```python
from build123d import *

# Parameters (mm, degrees)
SKETCH1_R           = 2.6035
BOSS_EXTRUDE1_DEPTH = 69.85


with BuildPart() as part:
    # Sketch1 → Boss-Extrude1 (new body)
    with BuildSketch(Plane(origin=(0, 0, 0), x_dir=(0, 0, -1), z_dir=(1, 0, 0))):
        with BuildLine():
            Line((6.333126718, -12.7), (9.550443118, -12.7))
            ThreePointArc((9.550443118, -12.7), (10.058366869, -12.192000006), (10.566443095, -12.699847501))
            ThreePointArc((10.566443095, -12.699847501), (12.082537762, -12.08250727), (12.699846982, -10.566399977))
            ThreePointArc((12.699846982, -10.566399977), (12.192000006, -10.058323491), (12.7, -9.5504))
            Line((12.7, -9.5504), (12.7, -6.3330836))
            ThreePointArc((12.7, -6.3330836), (12.192, -5.8250836), (12.7, -5.3170836))
            Line((12.7, -5.3170836), (12.7, -4.287469289))
            ThreePointArc((12.7, -4.287469289), (12.39275138, -3.545705502), (11.650987593, -3.238456882))
            Line((11.650987593, -3.238456882), (11.539212407, -3.238456882))
            ThreePointArc((11.539212407, -3.238456882), (10.79744862, -3.545705502), (10.4902, -4.287469289))
            Line((10.4902, -4.287469289), (10.4902, -6.402089023))
            ThreePointArc((10.4902, -6.402089023), (9.856505071, -7.351067942), (8.737131347, -7.129408934))
            Line((8.737131347, -7.129408934), (4.5085, -2.9104418))
            Line((4.5085, -2.9104418), (4.5085, 1.593185507))
            ThreePointArc((4.5085, 1.593185507), (4.750877967, 2.809883091), (5.441005833, 3.840816462))
            Line((5.441005833, 3.840816462), (8.737131347, 7.129408934))
            ThreePointArc((8.737131347, 7.129408934), (9.856505071, 7.351067942), (10.4902, 6.402089023))
            Line((10.4902, 6.402089023), (10.4902, 4.287469289))
            ThreePointArc((10.4902, 4.287469289), (10.79744862, 3.545705502), (11.539212407, 3.238456882))
            Line((11.539212407, 3.238456882), (11.650987593, 3.238456882))
            ThreePointArc((11.650987593, 3.238456882), (12.39275138, 3.545705502), (12.7, 4.287469289))
            Line((12.7, 4.287469289), (12.7, 5.3170836))
            ThreePointArc((12.7, 5.3170836), (12.192, 5.8250836), (12.7, 6.3330836))
            Line((12.7, 6.3330836), (12.7, 9.5504))
            ThreePointArc((12.7, 9.5504), (12.192000006, 10.058323491), (12.699846982, 10.566399977))
            ThreePointArc((12.699846982, 10.566399977), (12.082537762, 12.08250727), (10.566443095, 12.699847501))
            ThreePointArc((10.566443095, 12.699847501), (10.058366869, 12.192000006), (9.550443118, 12.7))
            Line((9.550443118, 12.7), (6.333126718, 12.7))
            ThreePointArc((6.333126718, 12.7), (5.825126718, 12.192), (5.317126718, 12.7))
            Line((5.317126718, 12.7), (4.287512407, 12.7))
            ThreePointArc((4.287512407, 12.7), (3.54574862, 12.39275138), (3.2385, 11.650987593))
            Line((3.2385, 11.650987593), (3.2385, 11.539212407))
            ThreePointArc((3.2385, 11.539212407), (3.54574862, 10.79744862), (4.287512407, 10.4902))
            Line((4.287512407, 10.4902), (6.476788598, 10.4902))
            ThreePointArc((6.476788598, 10.4902), (7.432222385, 9.85140422), (7.207036008, 8.724370562))
            Line((7.207036008, 8.724370562), (3.898272566, 5.423169045))
            ThreePointArc((3.898272566, 5.423169045), (2.869120213, 4.736787962), (1.655778399, 4.4958))
            Line((1.655778399, 4.4958), (-1.655778399, 4.4958))
            ThreePointArc((-1.655778399, 4.4958), (-2.869120213, 4.736787962), (-3.898272566, 5.423169045))
            Line((-3.898272566, 5.423169045), (-7.207036008, 8.724370562))
            ThreePointArc((-7.207036008, 8.724370562), (-7.432222385, 9.85140422), (-6.476788598, 10.4902))
            Line((-6.476788598, 10.4902), (-4.287512407, 10.4902))
            ThreePointArc((-4.287512407, 10.4902), (-3.54574862, 10.79744862), (-3.2385, 11.539212407))
            Line((-3.2385, 11.539212407), (-3.2385, 11.650987593))
            ThreePointArc((-3.2385, 11.650987593), (-3.54574862, 12.39275138), (-4.287512407, 12.7))
            Line((-4.287512407, 12.7), (-5.317126718, 12.7))
            ThreePointArc((-5.317126718, 12.7), (-5.825126718, 12.192), (-6.333126718, 12.7))
            Line((-6.333126718, 12.7), (-9.550443118, 12.7))
            ThreePointArc((-9.550443118, 12.7), (-10.058366869, 12.192000006), (-10.566443095, 12.699847501))
            ThreePointArc((-10.566443095, 12.699847501), (-12.082537762, 12.08250727), (-12.699846982, 10.566399977))
            ThreePointArc((-12.699846982, 10.566399977), (-12.192000006, 10.058323491), (-12.7, 9.5504))
            Line((-12.7, 9.5504), (-12.7, 6.3330836))
            ThreePointArc((-12.7, 6.3330836), (-12.192, 5.8250836), (-12.7, 5.3170836))
            Line((-12.7, 5.3170836), (-12.7, 4.287469289))
            ThreePointArc((-12.7, 4.287469289), (-12.39275138, 3.545705502), (-11.650987593, 3.238456882))
            Line((-11.650987593, 3.238456882), (-11.539212407, 3.238456882))
            ThreePointArc((-11.539212407, 3.238456882), (-10.79744862, 3.545705502), (-10.4902, 4.287469289))
            Line((-10.4902, 4.287469289), (-10.4902, 6.402089023))
            ThreePointArc((-10.4902, 6.402089023), (-9.856505071, 7.351067942), (-8.737131347, 7.129408934))
            Line((-8.737131347, 7.129408934), (-5.441005833, 3.840816462))
            ThreePointArc((-5.441005833, 3.840816462), (-4.750877967, 2.809883091), (-4.5085, 1.593185507))
            Line((-4.5085, 1.593185507), (-4.5085, -1.593185507))
            ThreePointArc((-4.5085, -1.593185507), (-4.750877967, -2.809883091), (-5.441005833, -3.840816462))
            Line((-5.441005833, -3.840816462), (-8.737131347, -7.129408934))
            ThreePointArc((-8.737131347, -7.129408934), (-9.856505071, -7.351067942), (-10.4902, -6.402089023))
            Line((-10.4902, -6.402089023), (-10.4902, -4.287469289))
            ThreePointArc((-10.4902, -4.287469289), (-10.79744862, -3.545705502), (-11.539212407, -3.238456882))
            Line((-11.539212407, -3.238456882), (-11.650987593, -3.238456882))
            ThreePointArc((-11.650987593, -3.238456882), (-12.39275138, -3.545705502), (-12.7, -4.287469289))
            Line((-12.7, -4.287469289), (-12.7, -5.3170836))
            ThreePointArc((-12.7, -5.3170836), (-12.192, -5.8250836), (-12.7, -6.3330836))
            Line((-12.7, -6.3330836), (-12.7, -9.5504))
            ThreePointArc((-12.7, -9.5504), (-12.192000006, -10.058323491), (-12.699846982, -10.566399977))
            ThreePointArc((-12.699846982, -10.566399977), (-12.082537762, -12.08250727), (-10.566443095, -12.699847501))
            ThreePointArc((-10.566443095, -12.699847501), (-10.058366869, -12.192000006), (-9.550443118, -12.7))
            Line((-9.550443118, -12.7), (-6.333126718, -12.7))
            ThreePointArc((-6.333126718, -12.7), (-5.825126718, -12.192), (-5.317126718, -12.7))
            Line((-5.317126718, -12.7), (-4.287512407, -12.7))
            ThreePointArc((-4.287512407, -12.7), (-3.54574862, -12.39275138), (-3.2385, -11.650987593))
            Line((-3.2385, -11.650987593), (-3.2385, -11.539212407))
            ThreePointArc((-3.2385, -11.539212407), (-3.54574862, -10.79744862), (-4.287512407, -10.4902))
            Line((-4.287512407, -10.4902), (-6.416408329, -10.4902))
            ThreePointArc((-6.416408329, -10.4902), (-7.41473083, -9.822813117), (-7.179650497, -8.645192506))
            Line((-7.179650497, -8.645192506), (-3.952270251, -5.423690499))
            ThreePointArc((-3.952270251, -5.423690499), (-2.922936451, -4.736929036), (-1.709253557, -4.4958))
            Line((-1.709253557, -4.4958), (1.709253557, -4.4958))
            ThreePointArc((1.709253557, -4.4958), (2.922936451, -4.736929036), (3.952270251, -5.423690499))
            Line((3.952270251, -5.423690499), (7.179650497, -8.645192506))
            ThreePointArc((7.179650497, -8.645192506), (7.41473083, -9.822813117), (6.416408329, -10.4902))
            Line((6.416408329, -10.4902), (4.287512407, -10.4902))
            ThreePointArc((4.287512407, -10.4902), (3.54574862, -10.79744862), (3.2385, -11.539212407))
            Line((3.2385, -11.539212407), (3.2385, -11.650987593))
            ThreePointArc((3.2385, -11.650987593), (3.54574862, -12.39275138), (4.287512407, -12.7))
            Line((4.287512407, -12.7), (5.317126718, -12.7))
            ThreePointArc((5.317126718, -12.7), (5.825126718, -12.192), (6.333126718, -12.7))
        make_face()
        Circle(SKETCH1_R, mode=Mode.SUBTRACT)
    extrude(amount=BOSS_EXTRUDE1_DEPTH)


solid = part.part
```
Work out the finished part from the listing and answer in its coordinate system (mm). A direction names the side the tool comes from. Give positions to 0.01 mm unless a question says otherwise; leave off trailing zeros. Loops run counter-clockwise (first coordinate to the right, second up) from the corner with the lowest first, then second, coordinate; pieces in that order, holes last. Notation, with made-up numbers: (58.5, -19.5) -> (110.5, -19.5) arc R36 ccw to (110.5, 15.5) -> close; hole circle Ø9 at (-1, -24.5). An arc over 180 degrees is marked (long way). Write item = value, one per line. Start each with the question number.
(1) Find section A-A on z = 0. Give the vertices of the cut face in (x, y).
(2) Find the intervals of material crossed by probe 1 along Y at (x, z) = (6.5, 2); probe 2 along Y at (x, z) = (48.5, -8.75); probe 3 along Z at (x, y) = (22.5, -9), in increasing order. Write a range as from..to.
(3) The mould has two halves that part along Z. Classify faces 3 (the flat face through (34, 8, -12.7)), 4 (the cylindrical face through (34.436, 7.344, 9.872)), 5 (the flat face through (34, 8, 12.7)): +Z half, -Z half, draft (parallel to the pull), parting line (faces both ways), or undercut.
(4) Find section B-B on y = 0. Give the vertices of the cut face in (x, z), and give its area (3 significant figures).
(5) Given pin 1 Ø0.6 at (x, y) = (35, 5.5) entering from -Z; pin 2 Ø1.4 at (x, y) = (52.5, -1.5) entering from -Z; pin 3 Ø2 at (x, y) = (14.5, 1) entering from +Z; pin 4 Ø1.7 at (x, z) = (48.5, 0.5) entering from +Y, each flat-ended and moving along its own axis, determine where each tip first touches the part or whether it passes through.
(6) Which of the six approach directions +Z, -Z, +X, -X, +Y, -Y give full straight-line access (tool end or side, diameter ignored) to faces 1 (the flat face through (34, 12.7, -8)), 2 (the flat face through (34, -10.49, -5))?
From the geometry:
q1.outline = (0, -4.5) -> (69.85, -4.5) -> (69.85, -2.6) -> (0, -2.6) -> close; (0, 2.6) -> (69.85, 2.6) -> (69.85, 4.5) -> (0, 4.5) -> close
q2.probe_1 = -4.51..-1.67, 1.67..4.51
q2.probe_2 = -12.7..-7.14, 7.14..12.7
q2.probe_3 = -12.7..-7.42, 7.42..12.7
q3.face_3 = -Z half
q3.face_4 = undercut
q3.face_5 = +Z half
q4.outline = (0, -4.51) -> (69.85, -4.51) -> (69.85, -2.6) -> (0, -2.6) -> close; (0, 2.6) -> (69.85, 2.6) -> (69.85, 4.51) -> (0, 4.51) -> close
q4.area = 266 mm^2
q5.pin_1 = -12.7
q5.pin_2 = -4.51
q5.pin_3 = 4.53
q5.pin_4 = 4.5
q6.face_1 = +Z, -Z, +X, -X, +Y
q6.face_2 = +X, -X
